The model under review builds one solid part; all positions refer to its coordinate system, in mm. Face numbers are marked on the shaded views. A direction names the side the tool comes from. Give positions to 0.01 mm unless a question says otherwise; leave off trailing zeros. Write each loop counter-clockwise with the first axis right and the second up, starting at its lowest first coordinate (ties: lowest second). Pieces come first, ordered by that corner, then holes. Notation, with made-up numbers: M 44,47.5 L 87,47.5 A35 ccw 87,84.5 Z; hole C -17,75.5 d9. An arc over 180 degrees is marked long. Write each question's results on one line, items separated by ' | '. Start each with the question number.
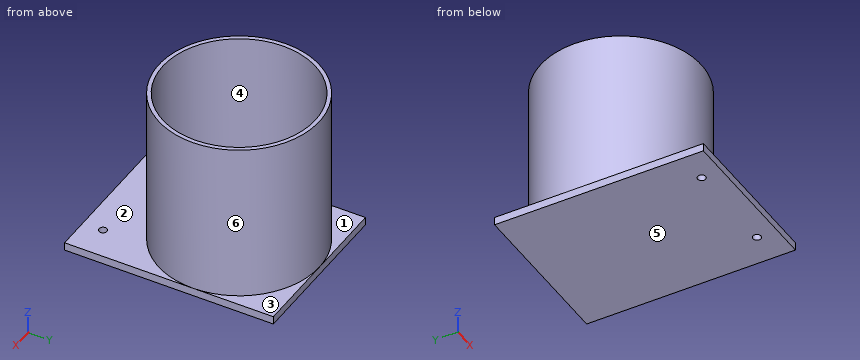
Autodesk Inventor part; units mm, degrees
ref_plane "YZ Plane" through (0, 0, 0) normal (1, 0, 0) x (0, 1, 0)
ref_plane "XZ Plane" through (0, 0, 0) normal (0, 1, 0) x (-1, 0, 0)
ref_plane "XY Plane" through (0, 0, 0) normal (0, 0, 1) x (1, 0, 0)
sketch "Sketch1" plane through (0, 0, 0) normal (0, 0, 1) x (1, 0, 0)
  line L0 (0, 0) -> (100, 0)
  line L1 (100, 0) -> (100, 130)
  line L2 (100, 130) -> (0, 130)
  line L3 (0, 130) -> (0, 0)
  dimension "d0" = 100
  dimension "d1" = 130
extrude "Extrusion1" add sketch "Sketch1" along normal blind 5
sketch "Sketch2" plane through (0, 0, 5) normal (0, 0, 1) x (1, 0, 0)
  line L0 (0, 130) -> (0, 0)
  line L1 (100, 130) -> (0, 130)
  line L2 (0, 0) -> (100, 0)
  line L3 (100, 0) -> (100, 130)
  line L4 (100, 130) -> (0, 130)
  line L5 (0, 130) -> (0, 0)
  circle A0 centre (50, 80) radius 50
  circle A1 centre (50, 80) radius 47.5
  dimension "d4" = 95
extrude "Extrusion2" add sketch "Sketch2" along normal blind 100 contours A0
sketch "Sketch3" plane through (0, 0, 5) normal (0, 0, 1) x (1, 0, 0)
  line L0 (100, 0) -> (100, 130)
  line L1 (0, 80) -> (0, 0)
  line L2 (100, 0) -> (0, 0)
  line L3 (0, 0) -> (0, 25)
  line L4 (0, 25) -> (100, 25)
  line L5 (100, 25) -> (100, 0)
  circle A0 centre (80, 12.5) radius 2.5
  circle A1 centre (20, 12.5) radius 2.5
  point P0 (0, 12.5)
  point P1 (100, 12.5)
  dimension "d7" = 25
  dimension "d8" = 5
  dimension "d9" = 5
  dimension "d10" = 20
  dimension "d11" = 20
  dimension "d12" = 12.5
  dimension "d13" = 12.5
extrude "Extrusion3" cut sketch "Sketch3" against normal blind 100 contours A0 | A1
thread "Thread1"
thread "Thread2"
properties part number "Reservoir"
(1) Wall thickness on L1, parallel to Y at x = 20, z = 1.05; L2, parallel to X at y = 12, z = 3; L3, parallel to Y at x = 50, z = 67: over which ranges is each line inside the solid? List them lowest first.
(2) Clearance check with flat-ended pins moving along their axes: P1, Ø6, axis at x = 60, y = 33.5, coming from the -Z side; P2, Ø4, axis at x = 20, y = 12.5, coming from the -Z side; P3, Ø10, axis at x = 68, z = 71.5, coming from the +Y side; P4, Ø8, axis at y = 114, z = 69.5, coming from the +X side. State where each tip first meets the part, or that it passes through.
(3) Add section B-B (y = 58). State the section outline as (x, z) points, then the cut area to 3 significant figures.
(4) Add section A-A (x = 80). State the section outline as (y, z) points, then the cut area to 3 significant figures.
(5) Add section C-C (z = 82.5). State the section outline as (x, y) points.
(6) Draft analysis for pull direction X (two halves, no side actions). For the marked faces 4, 5 and 6, state which applies: pulls with the +X half, pulls with the -X half, needs draft (parallel to the pull), parting line crosses it, or undercut.
(7) Machinability: for the marked faces 1, 2 and 3, which of the approach directions +Z, -Z, +X, -X, +Y, -Y give a long, thin tool a straight path to every point of the face, cutting with its end or side? Answer none if there is none.
(8) Add section D-D (x = 9.5). State the section outline as (y, z) points, then the cut area to 3 significant figures.
Calculated:
1) L1: y = 0 to 10, 15 to 130 | L2: x = 0 to 17.55, 22.45 to 77.55, 82.45 to 100 | L3: y = 30 to 32.5, 127.5 to 130
2) P1: stops at z = 0 | P2: passes through | P3: stops at y = 128.28 | P4: stops at x = 90
3) outline: M 0,0 L 100,0 L 100,5 L 94.9,5 L 94.9,105 L 92.1,105 L 92.1,5 L 7.9,5 L 7.9,105 L 5.1,105 L 5.1,5 L 0,5 Z | area: 1,060 mm²
4) outline: M 0,0 L 10,0 L 10,5 L 0,5 Z; M 15,0 L 130,0 L 130,5 L 120,5 L 120,105 L 116.83,105 L 116.83,5 L 43.17,5 L 43.17,105 L 40,105 L 40,5 L 15,5 Z | area: 1,260 mm²
5) outline: C 50,80 d100; hole C 50,80 d95
6) face 4: undercut | face 5: needs draft | face 6: parting line crosses it
7) face 1: +Z, -X, +Y | face 2: +Z, -Y | face 3: +Z, +X, +Y
8) outline: M 0,0 L 130,0 L 130,5 L 109.32,5 L 109.32,105 L 104.82,105 L 104.82,5 L 55.18,5 L 55.18,105 L 50.68,105 L 50.68,5 L 0,5 Z | area: 1,550 mm²
